Job drawing, mm, ordinate dimensions from the low corner. One solid piece. A direction names the side the tool comes from. Round coordinates to 2 decimals unless told otherwise and drop trailing zeros.
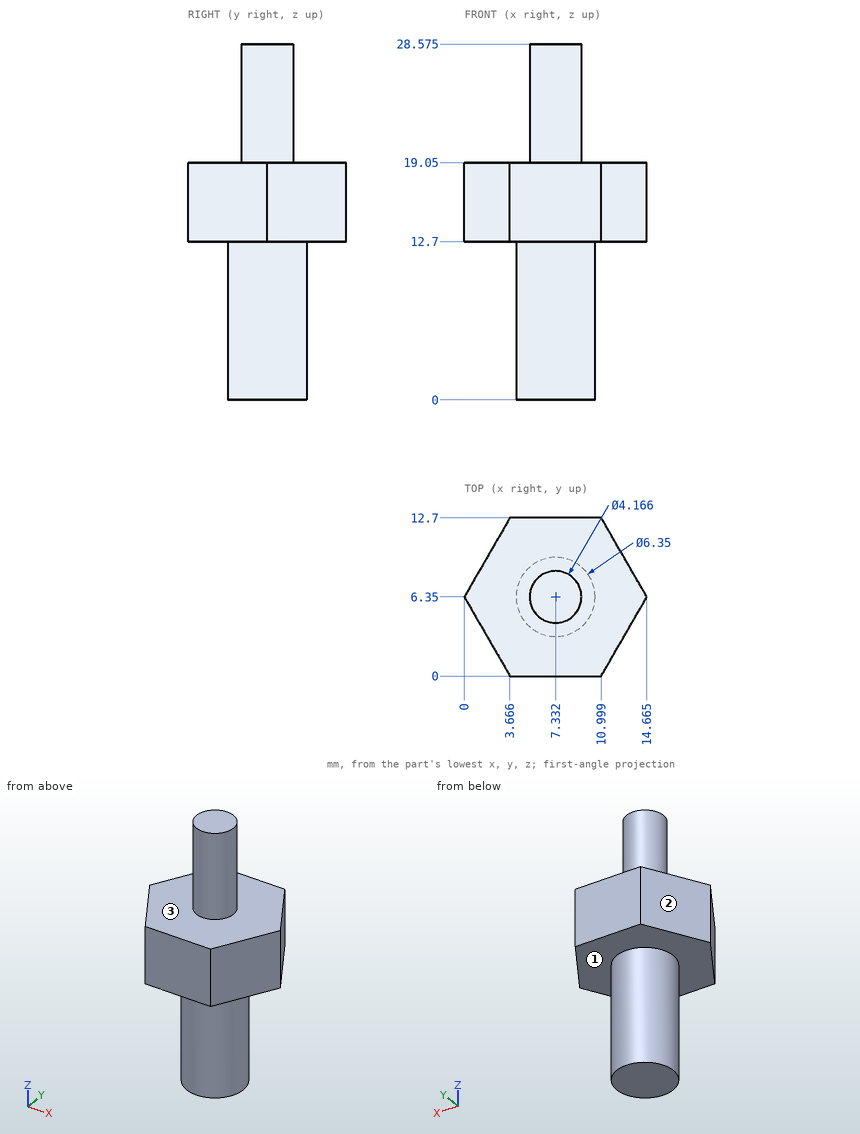
1) Drop flat-ended pins along their axis: pin 1 Ø8 at (x, z) = (11, 10) entering from -Y; pin 2 Ø1 at (y, z) = (10.5, 21) entering from +X; pin 3 Ø5 at (x, z) = (5.5, 4) entering from +Y (3 decimals); pin 4 Ø1 at (y, z) = (6.5, 7.5) entering from -X. Give the stop position or say it passes through.
Values:
pin 1: stops at y = 0
pin 2: passes through
pin 3: stops at y = 9.525
pin 4: stops at x = 4.16
2) Wall check: line 1 along X through (y, z) = (6.5, 2.5); line 2 along Z through (x, y) = (10.75, 11.5); line 3 along Y through (x, z) = (7.5, 25.5) (1 decimal). Give the ranges that are in metal, low to high.
Values:
line 1: x = 4.16 to 10.5
line 2: z = 12.7 to 19.05
line 3: y = 4.3 to 8.4
3) Tool access for the marked faces 1, 2 and 3: list every direction of +Z, -Z, +X, -X, +Y, -Y with a clear straight run to the whole face (end or side of a thin tool).
Values:
face 1: -Z
face 2: +Z, -Z, -X, +Y
face 3: +Z
